Source: CAD feature listing. Evaluate the final solid. Frame: model axes, mm. Face numbers are marked on the shaded views. A direction names the side the tool comes from. Give positions to 0.01 mm unless a question says otherwise; leave off trailing zeros. Loops run counter-clockwise (first coordinate to the right, second up) from the corner with the lowest first, then second, coordinate; pieces in that order, holes last. Notation, with made-up numbers: M 47.5,18.5 L 52.5,18.5 A9 ccw 52.5,27.5 Z; hole C 55.25,-31.5 d2. An arc over 180 degrees is marked long. Write item = value, one per line.
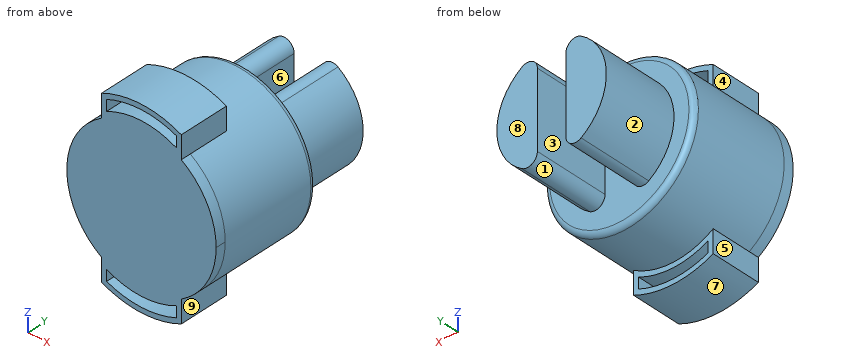
from build123d import *

# Parameters (mm, degrees)
SKETCH1_R           = 15
BOSS_EXTRUDE1_DEPTH = 20
SKETCH2_R           = 11
BOSS_EXTRUDE2_DEPTH = 15
SKETCH3_W           = 5.7
SKETCH3_H           = 24
CUT_EXTRUDE1_DEPTH  = 15
FILLET3_R           = 1
FILLET4_R           = 2
BOSS_EXTRUDE3_DEPTH = 2
BOSS_EXTRUDE4_START = -10
BOSS_EXTRUDE4_DEPTH = 10
CUT_EXTRUDE2_DEPTH  = 11
CUT_EXTRUDE3_DEPTH  = 11


with BuildPart() as part:
    # Sketch1 → Boss-Extrude1 (new body)
    with BuildSketch(Plane(origin=(0, 0, 0), x_dir=(1, 0, 0), z_dir=(0, 1, 0))):
        with Locations(Location((0, 0, 0), (0, 0, 270))):
            Circle(SKETCH1_R)
    extrude(amount=-BOSS_EXTRUDE1_DEPTH)

    # Sketch2 → Boss-Extrude2 (add)
    with BuildSketch(Plane(origin=(0, 0, 0), x_dir=(1, 0, 0), z_dir=(0, 1, 0))):
        with Locations(Location((0, 0, 0), (0, 0, 270))):
            Circle(SKETCH2_R)
    extrude(amount=BOSS_EXTRUDE2_DEPTH)

    # Sketch3 → Cut-Extrude1 (cut)
    with BuildSketch(Plane(origin=(0, 15, 0), x_dir=(1, 0, 0), z_dir=(0, 1, 0))):
        Rectangle(SKETCH3_W, SKETCH3_H)
    extrude(amount=-CUT_EXTRUDE1_DEPTH, mode=Mode.SUBTRACT)

    # Fillet3
    fillet3_edges = [part.edges().sort_by_distance(p)[0] for p in [
        (0, 0, -15),
    ]]
    fillet(fillet3_edges, radius=FILLET3_R)

    # Fillet4
    fillet4_edges = [part.edges().sort_by_distance(p)[0] for p in [
        (-2.85, 7.5, -10.624382335),
        (-2.85, 7.5, 10.624382335),
        (2.85, 7.5, 10.624382335),
        (2.85, 7.5, -10.624382335),
    ]]
    fillet(fillet4_edges, radius=FILLET4_R)

    # Sketch4 → Boss-Extrude3 (add)
    with BuildSketch(Plane.XZ.offset(20)):
        with BuildLine():
            ThreePointArc((8, 12.68857754), (0, 15), (-8, 12.68857754))
            Line((-8, 12.68857754), (-8, -12.68857754))
            ThreePointArc((-8, -12.68857754), (0, -15), (8, -12.68857754))
            Line((8, -12.68857754), (8, 12.68857754))
        make_face()
        with BuildLine():
            ThreePointArc((8, 17.23368794), (0, 19), (-8, 17.23368794))
            Line((-8, 17.23368794), (-8, 12.68857754))
            ThreePointArc((-8, 12.68857754), (0, 15), (8, 12.68857754))
            Line((8, 12.68857754), (8, 17.23368794))
        make_face()
        with BuildLine():
            Line((-8, -12.68857754), (-8, -17.23368794))
            ThreePointArc((-8, -17.23368794), (0, -19), (8, -17.23368794))
            Line((8, -17.23368794), (8, -12.68857754))
            ThreePointArc((8, -12.68857754), (0, -15), (-8, -12.68857754))
        make_face()
        with BuildLine():
            Line((-8, -12.68857754), (-8, 12.68857754))
            ThreePointArc((-8, 12.68857754), (-15, 0), (-8, -12.68857754))
        make_face()
        with BuildLine():
            ThreePointArc((15, 0), (13.133925537, 7.245688373), (8, 12.68857754))
            Line((8, 12.68857754), (8, -12.68857754))
            ThreePointArc((8, -12.68857754), (13.133925537, -7.245688373), (15, 0))
        make_face()
    extrude(amount=BOSS_EXTRUDE3_DEPTH)

    # Sketch7 → Boss-Extrude4 (add)
    with BuildSketch(Plane.XZ.offset(22).offset(BOSS_EXTRUDE4_START)):
        with BuildLine():
            Line((-8, -12.68857754), (-8, -17.23368794))
            ThreePointArc((-8, -17.23368794), (0, -19), (8, -17.23368794))
            Line((8, -17.23368794), (8, -12.68857754))
            ThreePointArc((8, -12.68857754), (0, -15), (-8, -12.68857754))
        make_face()
        with BuildLine():
            ThreePointArc((8, 17.23368794), (0, 19), (-8, 17.23368794))
            Line((-8, 17.23368794), (-8, 12.68857754))
            ThreePointArc((-8, 12.68857754), (0, 15), (8, 12.68857754))
            Line((8, 12.68857754), (8, 17.23368794))
        make_face()
    extrude(amount=BOSS_EXTRUDE4_DEPTH)

    # Sketch8 → Cut-Extrude2 (cut)
    with BuildSketch(Plane(origin=(0, -12, 0), x_dir=(1, 0, 0), z_dir=(0, 1, 0))):
        with BuildLine():
            Line((7, 14.38749457), (7, 16.583123952))
            ThreePointArc((7, 16.583123952), (0, 18), (-7, 16.583123952))
            Line((-7, 16.583123952), (-7, 14.38749457))
            ThreePointArc((-7, 14.38749457), (0, 16), (7, 14.38749457))
        make_face()
    extrude(amount=-CUT_EXTRUDE2_DEPTH, mode=Mode.SUBTRACT)

    # Sketch9 → Cut-Extrude3 (cut)
    with BuildSketch(Plane(origin=(0, -12, 0), x_dir=(1, 0, 0), z_dir=(0, 1, 0))):
        with BuildLine():
            Line((-7, -14.38749457), (-7, -16.583123952))
            ThreePointArc((-7, -16.583123952), (0, -18), (7, -16.583123952))
            Line((7, -16.583123952), (7, -14.38749457))
            ThreePointArc((7, -14.38749457), (0, -16), (-7, -14.38749457))
        make_face()
    extrude(amount=-CUT_EXTRUDE3_DEPTH, mode=Mode.SUBTRACT)


solid = part.part
1. Cut plane D-D, the plane x = 3.75. Count the separate pieces of the cut face and the enclosed holes in it, then the cut area to 3 significant figures.
Derived:
separate_pieces = 3
enclosed_holes = 0
area = 957 mm²
2. Material intervals for probe 1 along Y at (x, z) = (1.5, -1); probe 2 along X at (y, z) = (8, -8.5); probe 3 along X at (y, z) = (2, 0), sorted ascending. Write a range as from..to.
Derived:
probe_1 = -22..0
probe_2 = -6.98..-3.07, 3.07..6.98
probe_3 = -11..-2.85, 2.85..11
3. Cut plane C-C, the plane y = -18.5. Return the cut outline in (x, z).
Derived:
outline = M -8,-17.23 A19 ccw 8,-17.23 L 8,-12.69 A15 ccw 8,12.69 L 8,17.23 A19 ccw -8,17.23 L -8,12.69 A15 ccw -8,-12.69 Z; hole M -7,-16.58 A18 ccw 7,-16.58 L 7,-14.39 A16 cw -7,-14.39 Z; hole M -7,14.39 A16 cw 7,14.39 L 7,16.58 A18 ccw -7,16.58 Z
4. Pull-direction query (X, two-part tool) for the marked faces 6, 7, 8 and 9; classes: +X half, -X half, draft (parallel to the pull), parting line (faces both ways), or undercut.
Derived:
face_6 = undercut
face_7 = parting line
face_8 = draft
face_9 = +X half
5. Cut plane A-A, the plane y = 4. Return the cut outline in (x, z).
Derived:
outline = M -5.93,-9.27 A2 ccw -2.85,-7.58 L -2.85,7.58 A2 ccw -5.93,9.27 A11 ccw Z; M 2.85,-7.58 A2 ccw 5.93,-9.27 A11 ccw 5.93,9.27 A2 ccw 2.85,7.58 Z
6. Reachability of the marked faces 1, 2, 3, 4 and 5 from +Z, -Z, +X, -X, +Y, -Y: full face, straight path, thin tool, end or side. Return the list, or none.
Derived:
face_1 = -Z, +Y
face_2 = -X, +Y
face_3 = +Z, -Z, +Y
face_4 = +Z, -X, +Y, -Y
face_5 = -Z, -X, +Y, -Y
7. Cut plane B-B, the plane x = 0. Return the cut outline in (y, z), then the cut area to 3 significant figures.
Derived:
outline = M -22,-19 L -12,-19 L -12,-18 L -22,-18 Z; M -22,-16 L -12,-16 L -12,-15 L -1,-15 A1 ccw 0,-14 L 0,14 A1 ccw -1,15 L -12,15 L -12,16 L -22,16 Z; M -22,18 L -12,18 L -12,19 L -22,19 Z
area = 700 mm²
8. First-contact query: pin 1 Ø1.9 at (x, z) = (2, -17) entering from +Y; pin 2 Ø1.5 at (x, y) = (-12, -3) entering from -Z; pin 3 Ø8 at (x, y) = (6, 8.5) entering from -Z. Flat tips, straight axial feed; report the tip coordinate or a pass-through.
Derived:
pin_1 = -12
pin_2 = -9.92
pin_3 = -9.58
